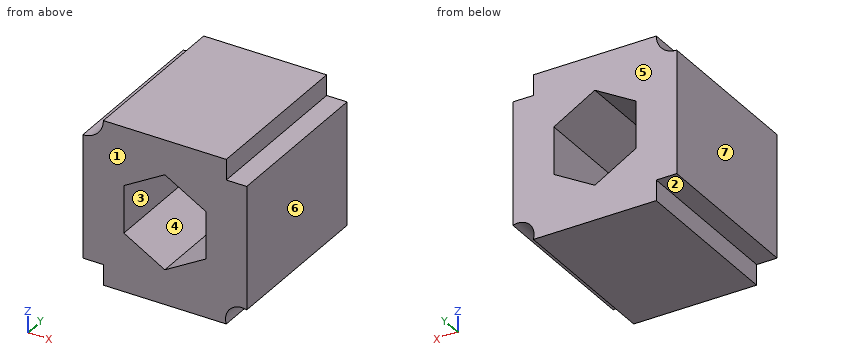
```python
from build123d import *

# Parameters (mm, degrees)
F1_DEPTH = 25.4


with BuildPart() as f1:
    # F0 (on Front) → F1 (new body)
    with BuildSketch(Plane.XZ):
        with BuildLine():
            Line((-9.525, -12.7), (9.525, -12.7))
            ThreePointArc((9.525, -12.7), (10.156475, -10.156475), (12.7, -9.525))
            Line((12.7, -9.525), (12.7, 9.525))
            Line((12.7, 9.525), (9.525, 9.516916))
            Line((9.525, 9.516916), (9.525, 12.7))
            Line((9.525, 12.7), (-9.525, 12.7))
            ThreePointArc((-9.525, 12.7), (-10.454936, 10.454936), (-12.7, 9.525))
            Line((-12.7, 9.525), (-12.7, -9.525))
            Line((-12.7, -9.525), (-9.525, -9.525))
            Line((-9.525, -9.525), (-9.525, -12.7))
        make_face()
        Polygon((6.35, 3.666174), (6.35, -3.666174), (0, -7.332348), (-6.35, -3.666174), (-6.35, 3.666174), (0, 7.332348), align=None, mode=Mode.SUBTRACT)
    extrude(amount=F1_DEPTH)


solid = f1.part
```
The listing builds one solid part. Answer for the finished solid, in the listing's coordinates (mm). Face numbers are marked on the shaded views. A direction names the side the tool comes from. Give positions to 0.01 mm unless a question says otherwise; leave off trailing zeros. Write each loop counter-clockwise with the first axis right and the second up, starting at its lowest first coordinate (ties: lowest second). Pieces come first, ordered by that corner, then holes. Notation, with made-up numbers: (77.5, 78) - (131.5, 78) arc R20 ccw to (131.5, 115) - close; hole circle Ø8 at (-30, 11.25). An arc over 180 degrees is marked (long way). Use one line per item in the form item = value. Start each with the question number.
1) A tool of negligible diameter and unlimited length cuts with its end or side. For the marked faces 1, 2 and 3, from which of +Z, -Z, +X, -X, +Y, -Y can it reach the whole face along a straight path? Write none if from no direction.
2) Find section C-C on x = -0.5. Determine the outline of the cut face in (y, z), plus the area to 3 significant figures.
3) Find section A-A on y = -15. Determine the outline of the cut face in (x, z) (3 decimals), plus the area to 3 significant figures.
4) Find section B-B on z = 3.25. Determine the outline of the cut face in (x, y).
5) The mould has two halves that part along X. Classify the marked faces 4, 5, 6 and 7: pulls with the +X half, pulls with the -X half, needs draft (parallel to the pull), parting line crosses it, or undercut.
6) Find section D-D on z = 10.5. Determine the outline of the cut face in (x, y) (3 decimals).
7) Consider line 1 along X through (y, z) = (-23.5, -3); line 2 along X through (y, z) = (-22, -6.5); line 3 along Z through (x, y) = (5, -23). Determine where each line is inside the solid, lowest interval first. Write a range as from..to.
8) Flat-ended cylindrical pins translate along their axes: pin 1 Ø1 at (y, z) = (-8, 11) entering from +X (3 decimals); pin 2 Ø1 at (y, z) = (-14, -11.5) entering from -X (3 decimals); pin 3 Ø1 at (x, y) = (-11, -18) entering from -Z (3 decimals); pin 4 Ø2 at (x, z) = (-5, -1) entering from +Y. Find the tip coordinate at first contact, or state that the pin passes through.
Geometry results:
q1.face_1 = +Z, -Z, +X, -X, -Y
q1.face_2 = -Z, -X, +Y, -Y
q1.face_3 = +Y, -Y
q2.outline = (-25.4, -12.7) - (0, -12.7) - (0, -7.04) - (-25.4, -7.04) - close; (-25.4, 7.04) - (0, 7.04) - (0, 12.7) - (-25.4, 12.7) - close
q2.area = 287 mm2
q3.outline = (-12.7, -9.525) - (-9.525, -9.525) - (-9.525, -12.7) - (9.525, -12.7) arc R2.54 cw to (12.7, -9.525) - (12.7, 9.525) - (9.525, 9.517) - (9.525, 12.7) - (-9.525, 12.7) arc R3.175 cw to (-12.7, 9.525) - close; hole (-6.35, -3.666) - (0, -7.332) - (6.35, -3.666) - (6.35, 3.666) - (0, 7.332) - (-6.35, 3.666) - close
q3.area = 468 mm2
q4.outline = (-12.7, -25.4) - (-6.35, -25.4) - (-6.35, 0) - (-12.7, 0) - close; (6.35, -25.4) - (12.7, -25.4) - (12.7, 0) - (6.35, 0) - close
q5.face_4 = undercut
q5.face_5 = needs draft
q5.face_6 = pulls with the +X half
q5.face_7 = pulls with the -X half
q6.outline = (-10.411, -25.4) - (9.525, -25.4) - (9.525, 0) - (-10.411, 0) - close
q7.line_1 = -12.7..-6.35, 6.35..12.7
q7.line_2 = -12.7..-1.44, 1.44..12.7
q7.line_3 = -12.7..-4.45, 4.45..12.7
q8.pin_1 = 9.525
q8.pin_2 = -9.525
q8.pin_3 = -9.525
q8.pin_4 = through
